Verification items for the finished model (mm, model axes). A direction names the side the tool comes from. Coordinates: 2 decimals unless noted, no trailing zeros. Write each loop counter-clockwise with the first axis right and the second up, starting at its lowest first coordinate (ties: lowest second). Pieces come first, ordered by that corner, then holes. Notation, with made-up numbers: (43, 38) -> (89, 38) arc R36 cw to (89, 77) -> close; hole circle Ø6 at (49, 60). An arc over 180 degrees is marked (long way). Write each question's results on one line, items separated by ' | '. Start each with the question number.
from build123d import *

# Parameters (mm, degrees)
F0_W          = 3
F0_H          = 4.5
F2_R          = 0.8
F3_DEPTH      = 25
F4_DEPTH      = 25
F4_DEPTH_BACK = 25
F5_R          = 1
F6_DEPTH      = 25


with BuildPart() as f1:
    # F0 (on Right) → F1 (revolve)
    with BuildSketch(Plane.YZ):
        Polygon((0, 4.5), (0, 0), (5.5, 0), (5.5, 4.5), (5.5, 7), (5, 7), (5, 4), (3.5, 4), (3.5, 7), (2, 7), (2, 4), (0.5, 4), (0.5, 7), (0, 7), align=None)
        with Locations((7, 2.25)):
            Rectangle(F0_W, F0_H)
        with Locations((-1.5, 2.25)):
            Rectangle(F0_W, F0_H)
    revolve(axis=Axis((0, 2.7052562218, 0), (0, 1, 0)))

    # F2 (on Top) → F3 (cut)
    with BuildSketch(Plane.XY):
        with Locations((0, 2.75)):
            Circle(F2_R)
    extrude(amount=-F3_DEPTH, mode=Mode.SUBTRACT)

    # F2 (on Top) → F4 (cut, two sides)
    with BuildSketch(Plane.XY) as f4_sk:
        with Locations((0, 2.75)):
            Circle(F2_R)
    extrude(amount=-F4_DEPTH, mode=Mode.SUBTRACT)
    extrude(f4_sk.sketch, amount=F4_DEPTH_BACK, mode=Mode.SUBTRACT)

    # F5 (on face) → F6 (cut)
    with BuildSketch(Plane.XZ.offset(3)):
        Circle(F5_R)
    extrude(amount=-F6_DEPTH, mode=Mode.SUBTRACT)


solid = f1.part
1. Sectioned sample at D-D on z = -4.25. Record the cut outline in (x, y).
2. Mould release check, pull along X, two halves, no side actions. Record for faces 1 (the flat face through (-5, 5.5, 0)), 2 (the cylindrical face through (0.763, 2.99, -3.752)), 3 (the cylindrical face through (1, 3, 0)), 4 (the cylindrical face through (-2.681, 0.246, 6.466)): +X half, -X half, draft (parallel to the pull), parting line (faces both ways), or undercut.
3. Material ranges on probe 1 along Y at (x, z) = (5.5, 4); probe 2 along Y at (x, z) = (0, 2.75); probe 3 along Y at (x, z) = (2.75, 3.5), recorded low to high. Write a range as from..to.
4. Sectioned sample at C-C on x = -4.25. Record the cut outline in (y, z).
5. Tool access check on faces 5 (the flat face through (4.4, 2, -0.1)), 6 (the flat face through (-3, 5, 3)), 7 (the cylindrical face through (4.46, 7.02, -0.59)), 8 (the flat face through (-5, 0, 0)). Record the directions out of +Z, -Z, +X, -X, +Y, -Y that give a thin tool (end or side, any length) a straight path to the whole face; none if there is none.
6. Sectioned sample at A-A on x = 0. State how many separate pieces and enclosed holes the cut face has, plus the area to 3 significant figures.
7. Depth check by flat-ended pin: pin 1 Ø2 at (x, y) = (0, 2.75) entering from +Z; pin 2 Ø3 at (x, y) = (-4.5, 3) entering from +Z; pin 3 Ø2 at (x, y) = (5, -1.5) entering from +Z. Enter the tip coordinate at first touch or a pass-through.
Computed values:
1) outline: (-5.56, 0) -> (-1.48, 0) -> (-1.48, -3) -> (1.48, -3) -> (1.48, 0) -> (5.56, 0) -> (5.56, 0.5) -> (-5.56, 0.5) -> close; (-5.56, 2) -> (-0.28, 2) arc R0.8 cw to (-0.28, 3.5) -> (-5.56, 3.5) -> close; (-5.56, 5) -> (5.56, 5) -> (5.56, 5.5) -> (1.48, 5.5) -> (1.48, 8.5) -> (-1.48, 8.5) -> (-1.48, 5.5) -> (-5.56, 5.5) -> close; (0.28, 2) -> (5.56, 2) -> (5.56, 3.5) -> (0.28, 3.5) arc R0.8 cw to start
2) face 1: draft | face 2: undercut | face 3: undercut | face 4: parting line
3) probe 1: y = 0..0.5, 2..3.5, 5..5.5 | probe 2: y = -3..1.95, 3.55..8.5 | probe 3: y = -3..0.5, 2..3.5, 5..8.5
4) outline: (-3, -1.48) -> (0, -1.48) -> (0, -5.56) -> (0.5, -5.56) -> (0.5, 5.56) -> (0, 5.56) -> (0, 1.48) -> (-3, 1.48) -> close; (2, -5.56) -> (3.5, -5.56) -> (3.5, 5.56) -> (2, 5.56) -> close; (5, -5.56) -> (5.5, -5.56) -> (5.5, -1.48) -> (8.5, -1.48) -> (8.5, 1.48) -> (5.5, 1.48) -> (5.5, 5.56) -> (5, 5.56) -> close
5) face 5: +X | face 6: none | face 7: +Y | face 8: -Y
6) separate pieces: 4 | enclosed holes: 0 | area: 71.4 mm^2
7) pin 1: stops at z = 6.99 | pin 2: stops at z = 6.32 | pin 3: stops at z = 2.06
